Design review of the part shown in the three views and the two pictorial views. Dimensions are in mm from the part's minimum x, y and z. A direction names the side the tool comes from. Round coordinates to 2 decimals unless told otherwise and drop trailing zeros. Loops run counter-clockwise (first coordinate to the right, second up) from the corner with the lowest first, then second, coordinate; pieces in that order, holes last. Notation, with made-up numbers: (-29, 60.5) - (1, 60.5) arc R17 cw to (1, 68.5) - close; hole circle Ø11 at (25, -7.75). An arc over 180 degrees is marked (long way). Return JSON: item names as keys, results as strings. Group by question number.
(1) We need section D-D, the plane z = 20. Write out the cut boundary in (x, y) (1 decimal).
(2) We need section C-C, the plane z = 4. Write out the cut boundary in (x, y) (1 decimal).
(3) Wall thickness on L1, parallel to X at y = 4.75, z = 9.5 (1 decimal); L2, parallel to Z at x = 7.25, y = 1.5: over which ranges is each line inside the solid? List them lowest first. Write a range as [from, to].
(4) Clearance check with flat-ended pins moving along their axes: pin 1 (1.5 mm diameter, centred on y = 2, z = 11, fed in from +X); pin 2 (4 mm diameter, centred on x = 5, y = 5.5, fed in from -Z); pin 3 (3 mm diameter, centred on x = 4.76, y = 4.76, fed in from -Z). State where each tip first meets the part, or that it passes through.
(5) We need section A-A, the plane x = 5.5. Write out the cut boundary in (y, z).
(6) The part is to be moulded in two halves that separate along X. For the marked faces 1, 2 and 3, say which applies: pulls with the +X half, pulls with the -X half, needs draft (parallel to the pull), parting line crosses it, or undercut.
(7) For the marked faces 4 and 5, list the 3-axis set-ups (+Z, -Z, +X, -X, +Y, -Y) from which the entire face can be reached by the end or side of a thin tool; tool diameter is ignored.
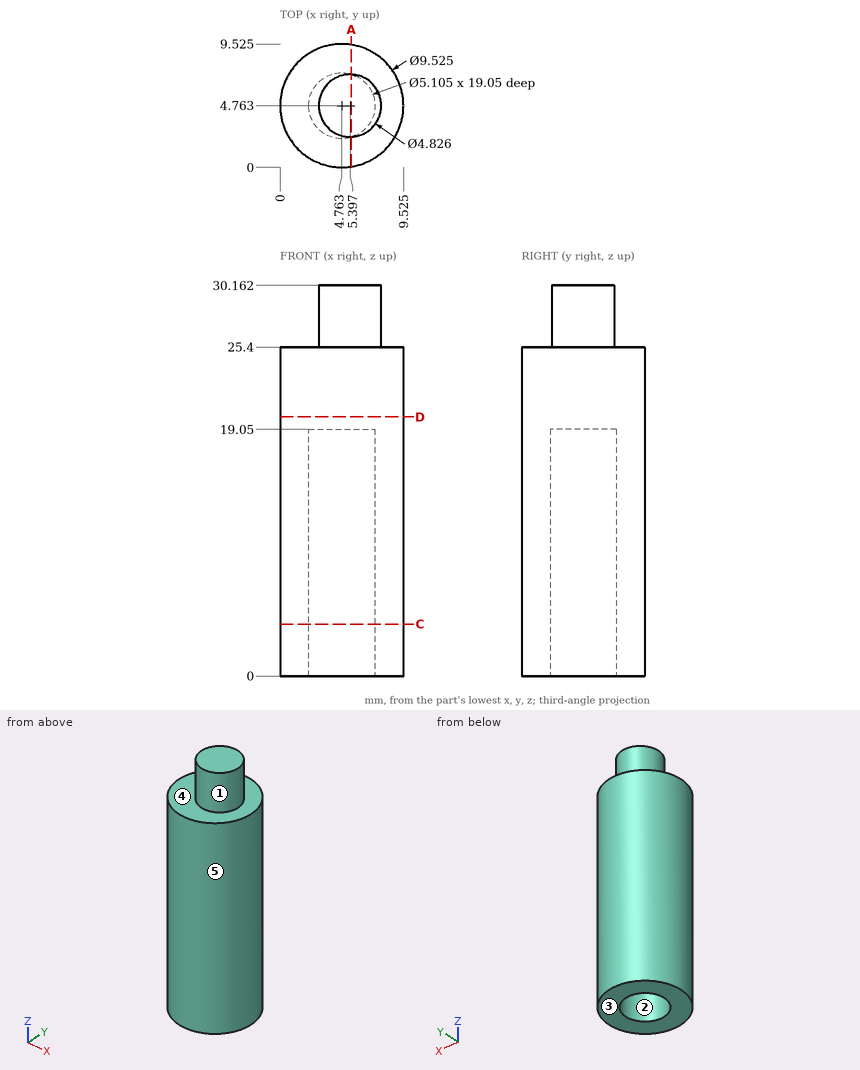
Solutions:
{
 "1": {"outline": "circle Ø9.5 at (4.8, 4.8)"},
 "2": {"outline": "circle Ø9.5 at (4.8, 4.8); hole circle Ø5.1 at (4.8, 4.8)"},
 "3": {"L1": "[0, 2.2], [7.3, 9.5]", "L2": "[0, 25.4]"},
 "4": {"pin 1": "x = 9.08", "pin 2": "z = 0", "pin 3": "z = 19.05"},
 "5": {"outline": "(0.06, 0) - (2.32, 0) - (2.32, 19.05) - (7.21, 19.05) - (7.21, 0) - (9.47, 0) - (9.47, 25.4) - (7.17, 25.4) - (7.17, 30.16) - (2.35, 30.16) - (2.35, 25.4) - (0.06, 25.4) - close"},
 "6": {"face 1": "parting line crosses it", "face 2": "undercut", "face 3": "needs draft"},
 "7": {"face 4": "+Z", "face 5": "+Z, -Z"}
}
